Check sheet for the modelled part. Datum: model origin and axes. Units: mm. Round coordinates to 2 decimals unless told otherwise and drop trailing zeros. Write each loop counter-clockwise with the first axis right and the second up, starting at its lowest first coordinate (ties: lowest second). Pieces come first, ordered by that corner, then holes.
Item 1: Cross-section at C-C on y = 17.78. Enter the section's corners in (x, z) (3 decimals), plus the area to 3 significant figures.
Item 2: Cross-section at A-A on x = 6.35. Enter the section's corners in (y, z) (3 decimals).
Item 3: Cross-section at B-B on z = 2.45. Enter the section's corners in (x, y) (3 decimals).
Item 4: Material ranges on line 1 (Y direction, x = 6.35, z = 0.7); line 2 (X direction, y = 17.78, z = 2.4); line 3 (Y direction, x = 6.5, z = 1.45), recorded low to high.
Item 5: Release check for a two-part mould opening along Y. For faces 1 (the cylindrical face through (7.119, 35.096, 1.565)), 2 (the flat face through (3, 19, 3.175)), 3 (the cylindrical face through (6.26, 8.38, 1.57)), 4 (the flat face through (6, 38.1, 2)) record: +Y half, -Y half, draft (parallel to the pull), parting line (faces both ways), or undercut.
Autodesk Inventor part; units mm, degrees
ref_plane "YZ Plane" through (0, 0, 0) normal (1, 0, 0) x (0, 1, 0)
ref_plane "XZ Plane" through (0, 0, 0) normal (0, 1, 0) x (-1, 0, 0)
ref_plane "XY Plane" through (0, 0, 0) normal (0, 0, 1) x (1, 0, 0)
sketch "Sketch1" plane through (0, 0, 0) normal (0, 0, 1) x (1, 0, 0)
  line L0 (0, 0) -> (12.7, 0)
  line L1 (12.7, 0) -> (12.7, 38.1)
  line L2 (12.7, 38.1) -> (0, 38.1)
  line L3 (0, 38.1) -> (0, 0)
  dimension "d0" = 12.7
  dimension "d1" = 38.1
extrude "Extrusion1" add sketch "Sketch1" along normal blind 3.175
sketch "Sketch2" plane through (0, 0, 3.175) normal (0, 0, 1) x (1, 0, 0)
  line L0 (0, 34.925) -> (6.35, 34.925)
  line L1 (12.7, 38.1) -> (0, 38.1)
  point P0 (6.35, 4.445)
  dimension "d23" = 3.175
hole "Hole1" at (6.35, 34.925, 3.175) direction (0, 0, -1) diameter 1.5748 end through all
sketch "Sketch3" plane through (0, 0, 3.175) normal (0, 0, 1) x (1, 0, 0)
  line L0 (12.7, 0) -> (12.7, 38.1)
  line L1 (0, 0) -> (12.7, 0)
  line L2 (0, 38.1) -> (0, 0)
  line L3 (0, 6.35) -> (6.35, 6.35)
  line L4 (6.35, 6.35) -> (6.35, 17.78)
  dimension "d24" = 6.35
  dimension "d25" = 6.35
  dimension "d26" = 11.43
hole "Hole3" at (6.35, 6.35, 3.175) at (6.35, 17.78, 3.175) direction (0, 0, -1) diameter 4.064 depth 25.4 tip angle 118
properties part number "ShoulderScrewHolderSlide"
Response values:
1. outline: (0, 0) - (4.318, 0) - (4.318, 3.175) - (0, 3.175) - close; (8.382, 0) - (12.7, 0) - (12.7, 3.175) - (8.382, 3.175) - close
1. area: 27.4 mm2
2. outline: (0, 0) - (4.318, 0) - (4.318, 3.175) - (0, 3.175) - close; (8.382, 0) - (15.748, 0) - (15.748, 3.175) - (8.382, 3.175) - close; (19.812, 0) - (34.138, 0) - (34.138, 3.175) - (19.812, 3.175) - close; (35.712, 0) - (38.1, 0) - (38.1, 3.175) - (35.712, 3.175) - close
3. outline: (0, 0) - (12.7, 0) - (12.7, 38.1) - (0, 38.1) - close; hole circle Ø4.064 at (6.35, 6.35); hole circle Ø4.064 at (6.35, 17.78); hole circle Ø1.575 at (6.35, 34.925)
4. line 1: y = 0 to 4.32, 8.38 to 15.75, 19.81 to 34.14, 35.71 to 38.1
4. line 2: x = 0 to 4.32, 8.38 to 12.7
4. line 3: y = 0 to 4.32, 8.38 to 15.75, 19.81 to 34.15, 35.7 to 38.1
5. face 1: undercut
5. face 2: draft
5. face 3: undercut
5. face 4: +Y half
